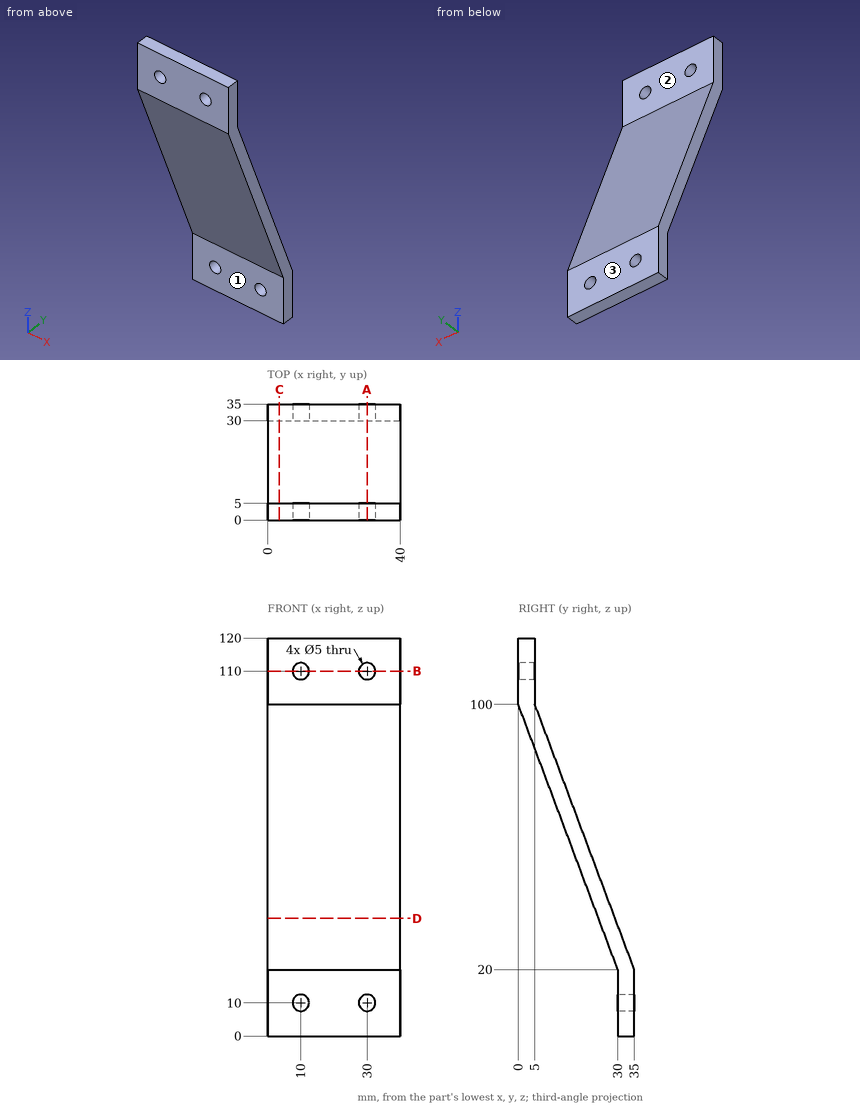
Job drawing, mm, ordinate dimensions from the low corner. One solid piece. A direction names the side the tool comes from. Coordinates: 2 decimals unless noted, no trailing zeros. Order: outer loops, then holes, each group sorted by start corner. A loop starts at its lowest first (then second) coordinate and runs counter-clockwise, first axis right, second up. Notation, with made-up numbers: M 61,-8.5 L 96,-8.5 A23 ccw 96,22.5 Z; hole C 2,78.25 d10. An arc over 180 degrees is marked long. Answer as CSV lines item,"result".
(1) Band-saw the part on C-C, the plane x = 3.5. List the corners of the cut face in (y, z), then the cut area to 3 significant figures.
Geometry says:
outline,"M 0,100 L 30,20 L 30,0 L 35,0 L 35,20 L 5,100 L 5,120 L 0,120 Z"
area,"600 mm2"
(2) Flat gauge pins, fed straight in: pin 1 (2 mm diameter, centred on x = 26, z = 74.5, fed in from +Y); pin 2 (1 mm diameter, centred on x = 35, z = 20, fed in from -Y); pin 3 (22 mm diameter, centred on x = 18.5, z = 106.5, fed in from +Y); pin 4 (6.5 mm diameter, centred on x = 10, z = 10, fed in from +Y). Where does each tip first touch, or does it go through?
Geometry says:
pin 1,"stops at y = 14.94"
pin 2,"stops at y = 29.81"
pin 3,"stops at y = 6.69"
pin 4,"stops at y = 35"
(3) Band-saw the part on A-A, the plane x = 30. List the corners of the cut face in (y, z).
Geometry says:
outline,"M 0,100 L 30,20 L 30,12.5 L 35,12.5 L 35,20 L 5,100 L 5,107.5 L 0,107.5 Z; M 0,112.5 L 5,112.5 L 5,120 L 0,120 Z; M 30,0 L 35,0 L 35,7.5 L 30,7.5 Z"
(4) Wall check: line 1 along Y through (x, z) = (18, 100.5); line 2 along Y through (x, z) = (27, 76). Give the ranges that are in metal, low to high.
Geometry says:
line 1,"y = 0 to 5"
line 2,"y = 9 to 14"
(5) Band-saw the part on B-B, the plane z = 110. List the corners of the cut face in (x, y).
Geometry says:
outline,"M 0,0 L 7.5,0 L 7.5,5 L 0,5 Z; M 12.5,0 L 27.5,0 L 27.5,5 L 12.5,5 Z; M 32.5,0 L 40,0 L 40,5 L 32.5,5 Z"
(6) Band-saw the part on D-D, the plane z = 35.5. List the corners of the cut face in (x, y), then the cut area to 3 significant figures.
Geometry says:
outline,"M 0,24.19 L 40,24.19 L 40,29.19 L 0,29.19 Z"
area,"200 mm2"
(7) 3-axis set-ups, long thin cutter, end or side, ignore diameter. For the marked faces 1, 2 and 3: which of +Z, -Z, +X, -X, +Y, -Y reach the whole face in a straight line?
Geometry says:
face 1,"-Z, +X, -X, -Y"
face 2,"+Z, +X, -X, +Y"
face 3,"+Z, -Z, +X, -X, +Y"
